from build123d import *

# Parameters (mm, degrees)
SKETCH_1_R          = 2
EXTRUDE_1_DEPTH     = 20
SKETCH_2_W          = 18
SKETCH_2_H          = 18
CUT_EXTRUDE_1_DEPTH = 102.724540869


with BuildPart() as part:
    # 草图1 → 凸台-拉伸1 (new body)
    with BuildSketch(Plane.XY):
        Polygon((5.657098919, 25.747533472), (25.657098919, 37.294538856), (25.657098919, -59.088008787), (5.657098919, -59.088008787), align=None)
        with Locations((15.657098919, 22.747533472)):
            Circle(SKETCH_1_R, mode=Mode.SUBTRACT)
        with Locations((15.657098919, 12.747533472)):
            Circle(SKETCH_1_R, mode=Mode.SUBTRACT)
        with Locations((15.657098919, -44.088008787)):
            Circle(SKETCH_1_R, mode=Mode.SUBTRACT)
        with Locations((15.657098919, -54.088008787)):
            Circle(SKETCH_1_R, mode=Mode.SUBTRACT)
    extrude(amount=EXTRUDE_1_DEPTH)

    # 草图2 → 切除-拉伸1 (cut, through all)
    with BuildSketch(Plane.XZ.offset(59.088008787)):
        with Locations((15.657098919, 10)):
            Rectangle(SKETCH_2_W, SKETCH_2_H)
    extrude(amount=-CUT_EXTRUDE_1_DEPTH, mode=Mode.SUBTRACT)


solid = part.part
Work out the finished part from the listing and answer in its coordinate system (mm). A direction names the side the tool comes from. Round coordinates to 2 decimals unless told otherwise and drop trailing zeros. Write each loop counter-clockwise with the first axis right and the second up, starting at its lowest first coordinate (ties: lowest second). Pieces come first, ordered by that corner, then holes.
1) A cutting plane is placed at D-D (x = 15.75). Give the number of separate pieces and of enclosed holes in the cut face, plus the area to 3 significant figures.
2) The mould has two halves that part along Y. Classify faces 1 (the cylindrical face through (15.397, -42.105, 19.493)), 2 (the flat face through (16, -12, 1)), 3 (the flat face through (16.4, -59.088, 19.6)): pulls with the +Y half, pulls with the -Y half, needs draft (parallel to the pull), parting line crosses it, or undercut.
3) A cutting plane is placed at B-B (x = 21.5). Give the vertices of the cut face in (y, z), plus the area to 3 significant figures.
4) A cutting plane is placed at A-A (z = 5). Give the vertices of the cut face in (x, y), plus the area to 3 significant figures.
5) Given pin 1 Ø8 at (x, z) = (18, 12) entering from +Y, flat-ended and moving along its own axis, determine where the tip first touches the part or whether it passes through.
6) A tool of negligible diameter and unlimited length cuts with its end or side. For faces 4 (the flat face through (24.657, -12, 10)), 5 (the flat face through (16, -10, 0)), from which of +Z, -Z, +X, -X, +Y, -Y can it reach the whole face along a straight path? Write none if from no direction.
7) A cutting plane is placed at C-C (y = -3). Give the vertices of the cut face in (x, z), plus the area to 3 significant figures.
8) Straight lines are drawn through the part: line 1 (X direction, y = 14.5, z = 16.75); line 2 (Z direction, x = 22.25, y = -45); line 3 (Y direction, x = 17, z = 19.25). For each, find the intervals that lie inside material, in ascending order.
Completed:
1. separate pieces: 10
1. enclosed holes: 0
1. area: 149 mm2
2. face 1: undercut
2. face 2: needs draft
2. face 3: pulls with the -Y half
3. outline: (-59.09, 0) - (34.89, 0) - (34.89, 1) - (-59.09, 1) - close; (-59.09, 19) - (34.89, 19) - (34.89, 20) - (-59.09, 20) - close
3. area: 188 mm2
4. outline: (5.66, -59.09) - (6.66, -59.09) - (6.66, 26.32) - (5.66, 25.75) - close; (24.66, -59.09) - (25.66, -59.09) - (25.66, 37.29) - (24.66, 36.72) - close
4. area: 181 mm2
5. pin 1: passes through
6. face 4: +Y, -Y
6. face 5: -Z, +X, -X, +Y, -Y
7. outline: (5.66, 0) - (25.66, 0) - (25.66, 20) - (5.66, 20) - close; hole (6.66, 1) - (24.66, 1) - (24.66, 19) - (6.66, 19) - close
7. area: 76.0 mm2
8. line 1: x = 5.66 to 6.66, 24.66 to 25.66
8. line 2: z = 0 to 1, 19 to 20
8. line 3: y = -59.09 to -55.57, -52.61 to -45.57, -42.61 to 11.27, 14.23 to 21.27, 24.23 to 32.3
